Print and shaded views of the part. All mm, measured from the part's lowest x, y and z. A direction names the side the tool comes from. Round coordinates to 2 decimals unless told otherwise and drop trailing zeros. Loops run counter-clockwise (first coordinate to the right, second up) from the corner with the lowest first, then second, coordinate; pieces in that order, holes last. Notation, with made-up numbers: (26, 21) - (65, 21) arc R27 ccw to (65, 47) - close; hole circle Ø5 at (4.25, 29.5). An arc over 180 degrees is marked (long way). Use one line per item in the form item = value.
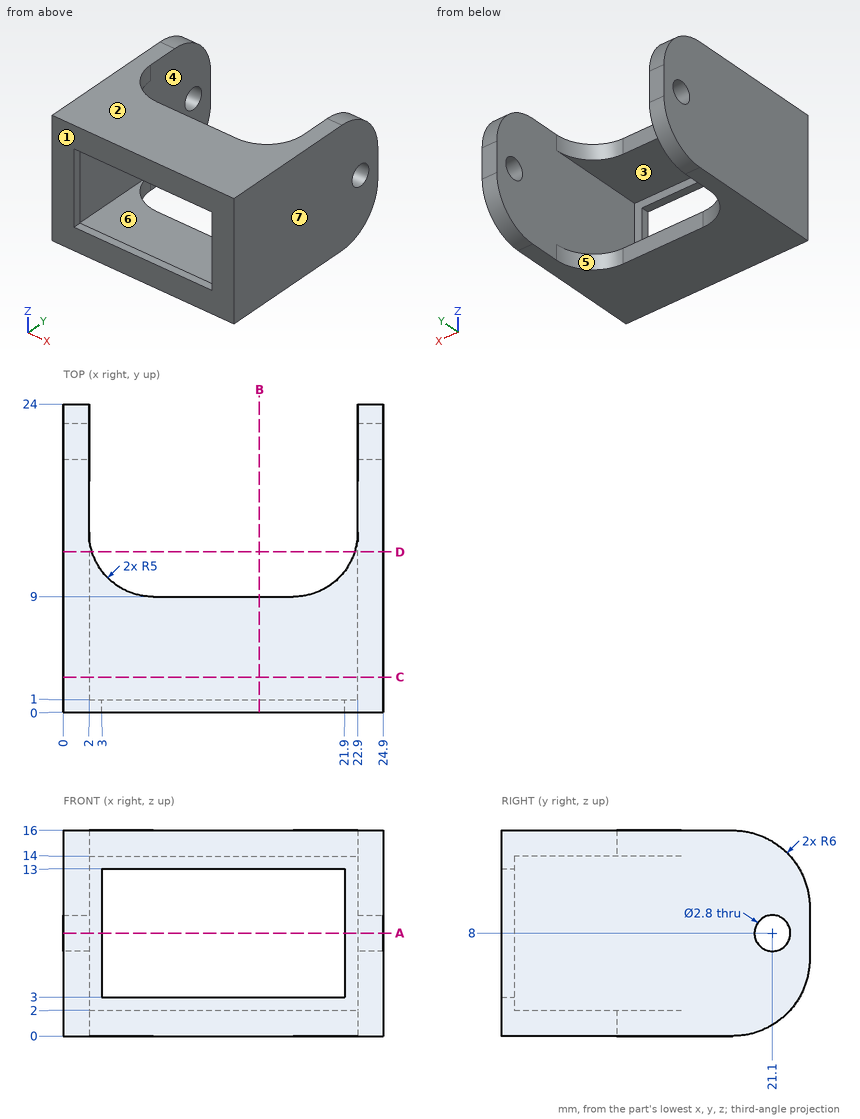
1. Cut at B-B, the plane x = 15.25. Give the cut face in (y, z), plus the area to 3 significant figures.
Geometry check:
outline = (0, 0) - (9, 0) - (9, 2) - (1, 2) - (1, 3) - (0, 3) - close; (0, 13) - (1, 13) - (1, 14) - (9, 14) - (9, 16) - (0, 16) - close
area = 38.0 mm^2
2. Cut at A-A, the plane z = 8. Give the cut face in (x, y).
Geometry check:
outline = (0, 0) - (3, 0) - (3, 1) - (2, 1) - (2, 19.7) - (0, 19.7) - close; (0, 22.5) - (2, 22.5) - (2, 24) - (0, 24) - close; (21.9, 0) - (24.9, 0) - (24.9, 19.7) - (22.9, 19.7) - (22.9, 1) - (21.9, 1) - close; (22.9, 22.5) - (24.9, 22.5) - (24.9, 24) - (22.9, 24) - close
3. Tool access for the marked faces 5, 6 and 7: list every direction of +Z, -Z, +X, -X, +Y, -Y with a clear straight run to the whole face (end or side of a thin tool).
Geometry check:
face_5 = +Z, -Z, +Y
face_6 = +Y
face_7 = +Z, -Z, +X, +Y, -Y
4. Wall check: probe 1 along X at (y, z) = (3.75, 9.5); probe 2 along Y at (x, z) = (23.7, 8); probe 3 along Z at (x, y) = (3, 3.25). Give the ranges that are in metal, low to high.
Geometry check:
probe_1 = 0 to 2, 22.9 to 24.9
probe_2 = 0 to 19.7, 22.5 to 24
probe_3 = 0 to 2, 14 to 16
5. Pull direction Z, two halves, no side cores. Call the marked faces 1, 2, 3 and 4: +Z half, -Z half, draft (parallel to the pull), parting line (faces both ways), or undercut.
Geometry check:
face_1 = draft
face_2 = +Z half
face_3 = undercut
face_4 = undercut
6. Cut at D-D, the plane y = 12.5. Give the cut face in (x, z), plus the area to 3 significant figures.
Geometry check:
outline = (0, 0) - (2.23, 0) - (2.23, 2) - (2, 2) - (2, 14) - (2.23, 14) - (2.23, 16) - (0, 16) - close; (22.67, 0) - (24.9, 0) - (24.9, 16) - (22.67, 16) - (22.67, 14) - (22.9, 14) - (22.9, 2) - (22.67, 2) - close
area = 65.8 mm^2
7. Cut at C-C, the plane y = 2.75. Give the cut face in (x, z), plus the area to 3 significant figures.
Geometry check:
outline = (0, 0) - (24.9, 0) - (24.9, 16) - (0, 16) - close; hole (2, 2) - (22.9, 2) - (22.9, 14) - (2, 14) - close
area = 148 mm^2
8. Flat gauge pins, fed straight in: pin 1 (1 mm diameter, centred on x = 13.5, z = 15, fed in from +Y); pin 2 (2 mm diameter, centred on y = 21.1, z = 8, fed in from -X); pin 3 (9.5 mm diameter, centred on x = 8.5, z = 10, fed in from +Y). Where does each tip first touch, or does it go through?
Geometry check:
pin_1 = 9
pin_2 = through
pin_3 = 9.11
